Input: part model. Units: mm. Frame: model coordinates. Face numbers are marked on the shaded views. A direction names the side the tool comes from. Coordinates: 2 decimals unless noted, no trailing zeros. Order: outer loops, then holes, each group sorted by start corner. A loop starts at its lowest first (then second) coordinate and runs counter-clockwise, first axis right, second up. Notation, with made-up numbers: (52.25, 58.25) -> (111.25, 58.25) arc R20 cw to (111.25, 75.25) -> close; hole circle Ø6 at (-28.75, 30). An arc over 180 degrees is marked (long way). Use one line per item in the form item = value. Start each with the question number.
1) Ray query, line 1 along Y through (x, z) = (-1.25, 7.5); line 2 along Z through (x, y) = (0.25, 67.5); line 3 along X through (y, z) = (40.5, 1.25). Return the intervals inside material, ascending.
2) Section query C-C on z = 8.5. Output: boundary loops of the cut face in (x, y).
3) Section query B-B on y = 55.5. Output: boundary loops of the cut face in (x, z) (3 decimals), then the cut area to 3 significant figures.
4) Access query for the marked faces 1 and 2. Directions: +Z, -Z, +X, -X, +Y, -Y. A direction counts if a zero-diameter tool reaches every point of the face in a straight line with its end or side. Return the directions, or none.
5) Pin query (flat end, axial travel): pin 1 (4 mm diameter, centred on y = 38, z = 6, fed in from +X); pin 2 (0.8 mm diameter, centred on y = 104, z = -1, fed in from -X); pin 3 (12 mm diameter, centred on x = 2.5, y = 58.5, fed in from +Z) (3 decimals); pin 4 (1.4 mm diameter, centred on x = 0, z = 1.5, fed in from +Y). Return the tip coordinate at first contact, or that it passes through.
6) Section query A-A on z = 0. Output: boundary loops of the cut face in (x, y) (3 decimals), then the cut area to 3 significant figures.
from build123d import *

# Parameters (mm, degrees)
FILLET1_R                       = 4
CUT_EXTRUDE3_DEPTH              = 106.978541224
CUT_EXTRUDE3_DEPTH_BACK         = 106.978541224
SKETCH4_W                       = 1.7
SKETCH4_H                       = 1.7
F_1_16_0_0625_DOWEL_HOLE1_D     = 1.5875
F_1_16_0_0625_DOWEL_HOLE1_DEPTH = 6
F_1_16_0_0625_DOWEL_HOLE1_TIP   = 0.476933116


with BuildPart() as part:
    # Sketch1 → Revolve1 (revolve)
    with BuildSketch(Plane.XY, mode=Mode.PRIVATE) as revolve1_sk:
        Polygon((0, 0), (10.16, 0), (10.16, 2.5), (3.175, 2.5), (3.175, 105), (0, 105), align=None)
    revolve(revolve1_sk.sketch.rotate(Axis((0, -31.831703756, 0), (0, 1, 0)), 90), axis=Axis((0, -31.831703756, 0), (0, 1, 0)))

    # Fillet1
    fillet1_edges = [part.edges().sort_by_distance(p)[0] for p in [
        (0, 2.5, 3.175),
    ]]
    fillet(fillet1_edges, radius=FILLET1_R)

    # Sketch4 → Cut-Extrude3 (cut, two sides: drawn at the far end of the back side and taken through both)
    with BuildSketch(Plane.XY.offset(-CUT_EXTRUDE3_DEPTH_BACK)):
        with Locations((0, 104.15)):
            Rectangle(SKETCH4_W, SKETCH4_H)
    extrude(amount=CUT_EXTRUDE3_DEPTH + CUT_EXTRUDE3_DEPTH_BACK, mode=Mode.SUBTRACT)

    # 1/16 (0.0625) Dowel Hole1
    with Locations(Plane(origin=(0, 0, 0), x_dir=(-1, 0, 0), z_dir=(0, -1, 0))):
        with Locations((5.675039265, -6.764822935), (-5.675039265, 6.764822935)):
            Hole(F_1_16_0_0625_DOWEL_HOLE1_D / 2, depth=F_1_16_0_0625_DOWEL_HOLE1_DEPTH)
            with Locations((0, 0, -(F_1_16_0_0625_DOWEL_HOLE1_DEPTH + F_1_16_0_0625_DOWEL_HOLE1_TIP / 2))):  # 118° drill point
                Cone(0, F_1_16_0_0625_DOWEL_HOLE1_D / 2, F_1_16_0_0625_DOWEL_HOLE1_TIP, mode=Mode.SUBTRACT)


solid = part.part
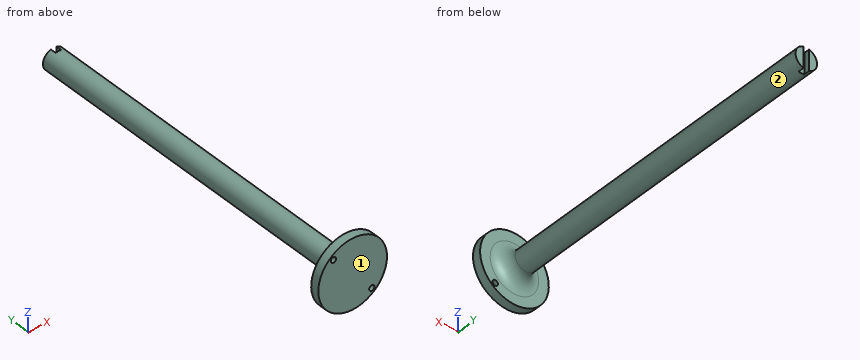
Answers below:
q1.line_1 = 0 to 2.5
q1.line_2 = -3.17 to 3.17
q1.line_3 = -2.92 to 2.92
q2.outline = (-5.57, 0) -> (5.57, 0) -> (5.57, 2.5) -> (-5.57, 2.5) -> close
q3.outline = circle Ø6.35 at (0, 0)
q3.area = 31.7 mm^2
q4.face_1 = +Z, -Z, +X, -X, -Y
q4.face_2 = +Y
q5.pin_1 = through
q5.pin_2 = -3.12
q5.pin_3 = 3.175
q5.pin_4 = 103.3
q6.outline = (-10.16, 0) -> (10.16, 0) -> (10.16, 2.5) -> (7.175, 2.5) arc R4 cw to (3.175, 6.5) -> (3.175, 105) -> (0.85, 105) -> (0.85, 103.3) -> (-0.85, 103.3) -> (-0.85, 105) -> (-3.175, 105) -> (-3.175, 6.5) arc R4 cw to (-7.175, 2.5) -> (-10.16, 2.5) -> close
q6.area = 706 mm^2
